```python
from build123d import *

# Parameters (mm, degrees)
SKETCH1_W           = 160
SKETCH1_H           = 200
BOSS_EXTRUDE1_DEPTH = 3
SKETCH2_R           = 1.5
SKETCH2_W           = 25
SKETCH2_H           = 2.05
SKETCH2_W_2         = 2
SKETCH2_H_2         = 50
SKETCH2_W_3         = 2.02
SKETCH2_H_3         = 30
SKETCH2_W_4         = 15
SKETCH2_H_4         = 15
SKETCH2_W_5         = 42
SKETCH2_W_6         = 4
SKETCH2_H_5         = 22
SKETCH2_W_7         = 3.05
SKETCH2_H_6         = 35
CUT_EXTRUDE1_DEPTH  = 3
SKETCH3_R           = 1.5
CUT_EXTRUDE2_DEPTH  = 129.097619025
SKETCH4_R           = 7.5
SKETCH4_R_2         = 1.5
SKETCH4_W           = 10
SKETCH4_H           = 80
SKETCH4_W_2         = 70
SKETCH4_H_2         = 10
CUT_EXTRUDE3_DEPTH  = 3
SKETCH5_R           = 1.5
CUT_EXTRUDE4_DEPTH  = 10


with BuildPart() as part:
    # Sketch1 → Boss-Extrude1 (new body)
    with BuildSketch(Plane(origin=(0, 0, 0), x_dir=(1, 0, 0), z_dir=(0, 1, 0))):
        Rectangle(SKETCH1_W, SKETCH1_H)
    extrude(amount=BOSS_EXTRUDE1_DEPTH)

    # Sketch2 → Cut-Extrude1 (cut)
    with BuildSketch(Plane(origin=(0, 3, 0), x_dir=(1, 0, 0), z_dir=(0, 1, 0))):
        with Locations(Location((-60, -90, 0), (0, 0, 270))):
            Circle(SKETCH2_R)
        with Locations(Location((60, -90, 0), (0, 0, 90))):
            Circle(SKETCH2_R)
        with Locations(Location((0, -10, 0), (0, 0, 270))):
            Circle(SKETCH2_R)
        with Locations(Location((-65, 70, 0), (0, 0, 270))):
            Circle(SKETCH2_R)
        with Locations(Location((65, 70, 0), (0, 0, 90))):
            Circle(SKETCH2_R)
        with Locations((27.5, -93.975)):
            Rectangle(SKETCH2_W, SKETCH2_H)
        with Locations((-27.5, -93.975)):
            Rectangle(SKETCH2_W, SKETCH2_H)
        with Locations((64.5, 0)):
            Rectangle(SKETCH2_W_2, SKETCH2_H_2)
        with Locations((-64.5, 0)):
            Rectangle(SKETCH2_W_2, SKETCH2_H_2)
        with Locations((71.99, 80)):
            Rectangle(SKETCH2_W_3, SKETCH2_H_3)
        with Locations((-30.5, 92.5)):
            Rectangle(SKETCH2_W_4, SKETCH2_H_4)
        with Locations((2, 93.975)):
            Rectangle(SKETCH2_W_5, SKETCH2_H)
        with Locations((-71.99, 80)):
            Rectangle(SKETCH2_W_3, SKETCH2_H_3)
        with Locations((-8, 60)):
            Rectangle(SKETCH2_W_6, SKETCH2_H_5)
        with Locations((13.525, 58.5)):
            Rectangle(SKETCH2_W_7, SKETCH2_H_6)
    extrude(amount=-CUT_EXTRUDE1_DEPTH, mode=Mode.SUBTRACT)

    # Sketch3 → Cut-Extrude2 (cut, through all)
    with BuildSketch(Plane(origin=(0, 3, 0), x_dir=(1, 0, 0), z_dir=(0, 1, 0))):
        with Locations(Location((-24.13, 27.6, 0), (0, 0, 270))):
            Circle(SKETCH3_R)
        with Locations(Location((24.13, 26.36, 0), (0, 0, 270))):
            Circle(SKETCH3_R)
        with Locations(Location((-24.13, -54.92, 0), (0, 0, 270))):
            Circle(SKETCH3_R)
        with Locations(Location((24.13, -48.57, 0), (0, 0, 270))):
            Circle(SKETCH3_R)
    extrude(amount=-CUT_EXTRUDE2_DEPTH, mode=Mode.SUBTRACT)

    # Sketch4 → Cut-Extrude3 (cut)
    with BuildSketch(Plane(origin=(0, 3, 0), x_dir=(1, 0, 0), z_dir=(0, 1, 0))):
        with Locations(Location((-45, 60, 0), (0, 0, 270))):
            Circle(SKETCH4_R)
        with Locations(Location((45, 60, 0), (0, 0, 90))):
            Circle(SKETCH4_R)
        with Locations(Location((-60, 87, 0), (0, 0, 270))):
            Circle(SKETCH4_R_2)
        with Locations(Location((60, 87, 0), (0, 0, 90))):
            Circle(SKETCH4_R_2)
        with Locations(Location((-65, 36, 0), (0, 0, 270))):
            Circle(SKETCH4_R_2)
        with Locations(Location((65, 36, 0), (0, 0, 90))):
            Circle(SKETCH4_R_2)
        with Locations((-45, -10)):
            Rectangle(SKETCH4_W, SKETCH4_H)
        with Locations((45, -10)):
            Rectangle(SKETCH4_W, SKETCH4_H)
        with Locations((0, -78)):
            Rectangle(SKETCH4_W_2, SKETCH4_H_2)
    extrude(amount=-CUT_EXTRUDE3_DEPTH, mode=Mode.SUBTRACT)

    # Sketch5 → Cut-Extrude4 (cut)
    with BuildSketch(Plane(origin=(0, 3, 0), x_dir=(1, 0, 0), z_dir=(0, 1, 0))):
        with Locations(Location((-74, -80, 0), (0, 0, 270))):
            Circle(SKETCH5_R)
        with Locations(Location((-74, -56, 0), (0, 0, 270))):
            Circle(SKETCH5_R)
        with Locations(Location((-45, -80, 0), (0, 0, 270))):
            Circle(SKETCH5_R)
        with Locations(Location((-45, -56, 0), (0, 0, 270))):
            Circle(SKETCH5_R)
        with Locations(Location((45, -80, 0), (0, 0, 270))):
            Circle(SKETCH5_R)
        with Locations(Location((45, -56, 0), (0, 0, 270))):
            Circle(SKETCH5_R)
        with Locations(Location((74, -80, 0), (0, 0, 270))):
            Circle(SKETCH5_R)
        with Locations(Location((74, -56, 0), (0, 0, 270))):
            Circle(SKETCH5_R)
    extrude(amount=-CUT_EXTRUDE4_DEPTH, mode=Mode.SUBTRACT)


solid = part.part
```
Check sheet for the modelled part. Datum: model origin and axes. Units: mm. Round coordinates to 2 decimals unless told otherwise and drop trailing zeros. Loops run counter-clockwise (first coordinate to the right, second up) from the corner with the lowest first, then second, coordinate; pieces in that order, holes last. Notation, with made-up numbers: (30.25, 65.5) -> (85.25, 65.5) arc R22 ccw to (85.25, 98.5) -> close; hole circle Ø10 at (37.25, 38.5). An arc over 180 degrees is marked (long way). Answer in a Markdown table with one row per item.
Q1. Sectioned sample at A-A on x = 32.5. Enter the section's corners in (y, z).
Data:
| item | result |
|---|---|
| outline | (0, -100) -> (3, -100) -> (3, 73) -> (0, 73) -> close; (0, 83) -> (3, 83) -> (3, 92.95) -> (0, 92.95) -> close; (0, 95) -> (3, 95) -> (3, 100) -> (0, 100) -> close |
Q2. Sectioned sample at D-D on z = 38.5. Enter the section's corners in (x, y).
Data:
| item | result |
|---|---|
| outline | (-80, 0) -> (-50, 0) -> (-50, 3) -> (-80, 3) -> close; (-40, 0) -> (40, 0) -> (40, 3) -> (-40, 3) -> close; (50, 0) -> (80, 0) -> (80, 3) -> (50, 3) -> close |
Q3. Release check for a two-part mould opening along X. For faces 1 (the face through (-1, 0, -1)), 2 (the face through (-52.32, 1.52, -61.63)) record: released by +X, released by -X, zero draft, split by the parting line, or undercut.
Data:
| item | result |
|---|---|
| face 1 | zero draft |
| face 2 | undercut |
Q4. Go/stop test with flat-tipped pins: P1, Ø1.5, axis at x = -32.5, y = 2, coming from the -Z side; P2, Ø2.5, axis at x = -24.13, z = -27.6, coming from the -Y side. Record where each tip stops, or that it passes through.
Data:
| item | result |
|---|---|
| P1 | stops at z = -85 |
| P2 | passes through |
Q5. Sectioned sample at C-C on z = -12.5. Enter the section's corners in (x, y), then the cut area to 3 significant figures.
Data:
| item | result |
|---|---|
| outline | (-80, 0) -> (-65.5, 0) -> (-65.5, 3) -> (-80, 3) -> close; (-63.5, 0) -> (-50, 0) -> (-50, 3) -> (-63.5, 3) -> close; (-40, 0) -> (40, 0) -> (40, 3) -> (-40, 3) -> close; (50, 0) -> (63.5, 0) -> (63.5, 3) -> (50, 3) -> close; (65.5, 0) -> (80, 0) -> (80, 3) -> (65.5, 3) -> close |
| area | 408 mm^2 |
Q6. Sectioned sample at B-B on z = 76. Enter the section's corners in (x, y), then the cut area to 3 significant figures.
Data:
| item | result |
|---|---|
| outline | (-80, 0) -> (-35, 0) -> (-35, 3) -> (-80, 3) -> close; (35, 0) -> (80, 0) -> (80, 3) -> (35, 3) -> close |
| area | 270 mm^2 |
Q7. Thickness scan on L1, parallel to X at y = 1.85, z = 30.5; L2, parallel to X at y = 1.4, z = -87; L3, parallel to X at y = 0.3, z = 23. Record the ranges inside material, lowest first.
Data:
| item | result |
|---|---|
| L1 | x = -80 to -50, -40 to 40, 50 to 80 |
| L2 | x = -80 to -73, -70.98 to -61.5, -58.5 to -38, -23 to 58.5, 61.5 to 70.98, 73 to 80 |
| L3 | x = -80 to -65.5, -63.5 to -50, -40 to 40, 50 to 63.5, 65.5 to 80 |
